Input: part model. Units: mm. Frame: model coordinates. Face numbers are marked on the shaded views. A direction names the side the tool comes from. Give positions to 0.01 mm unless a question says otherwise; leave off trailing zeros. Loops run counter-clockwise (first coordinate to the right, second up) from the corner with the lowest first, then second, coordinate; pieces in that order, holes last. Notation, with made-up numbers: (37, 40.25) -> (55, 40.25) arc R14 ccw to (55, 48.25) -> close; hole circle Ø11 at (-24, -9). An arc over 180 degrees is marked (long way). Answer as a JSON object with one key per item and string values. Group by question number.
```python
from build123d import *

# Parameters (mm, degrees)
F2_R     = 0.7
F3_DEPTH = 2.761
F4_R     = 0.25
F5_DEPTH = 0.751
F6_R     = 0.12


with BuildPart() as f1:
    # F0 (on Top) → F1 (revolve)
    with BuildSketch(Plane.XY):
        Polygon((0, 2.76), (0, 0), (1.065, 0), (1.065, 2.01), (2.75, 2.01), (2.75, 2.76), align=None)
    revolve(axis=Axis((0, 1.38, 0), (0, 1, 0)))

    # F2 (on face) → F3 (cut, through all)
    with BuildSketch(Plane.XZ):
        Circle(F2_R)
    extrude(amount=-F3_DEPTH, mode=Mode.SUBTRACT)

    # F4 (on face) → F5 (cut, through all)
    with BuildSketch(Plane.XZ.offset(-2.01)):
        with Locations((0, 2.12)):
            Circle(F4_R)
        with Locations((2.12, 0)):
            Circle(F4_R)
        with Locations((0, -2.12)):
            Circle(F4_R)
        with Locations((-2.12, 0)):
            Circle(F4_R)
    extrude(amount=-F5_DEPTH, mode=Mode.SUBTRACT)

    # F6
    f6_edges = [f1.edges().sort_by_distance(p)[0] for p in [
        (-2.75, 2.01, 0),
        (-1.065, 2.01, 0),
        (-1.065, 0, 0),
    ]]
    fillet(f6_edges, radius=F6_R)


solid = f1.part
```
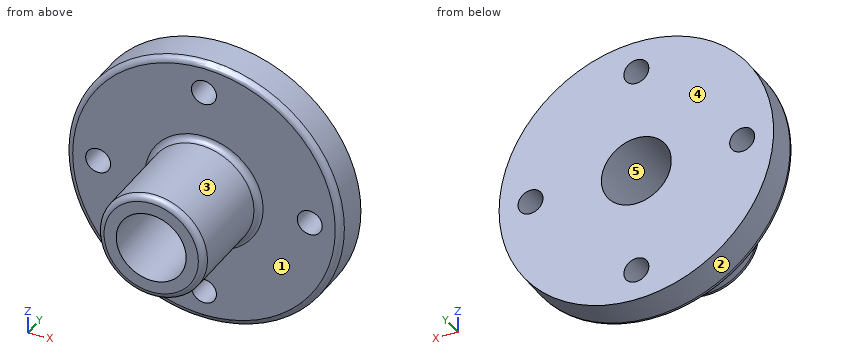
Q1. Pull-direction query (Z, two-part tool) for the marked faces 3, 4 and 5; classes: +Z half, -Z half, draft (parallel to the pull), parting line (faces both ways), or undercut.
Q2. Set-up query: the marked faces 1 and 2. Return all of +Z, -Z, +X, -X, +Y, -Y with unobstructed straight access to the full face (end or side cutting, diameter ignored); none if empty.
Q3. Section C-C on y = 1.05. Return the cut outline in (x, z) (3 decimals), then the cut area to 3 significant figures.
Q4. Ray query, probe 1 along Z at (x, y) = (0, 2.3); probe 2 along Z at (x, y) = (0, 1.3) (3 decimals); probe 3 along Y at (x, z) = (1.2, -2.35). Return the intervals inside material, ascending.
Q5. Section B-B on z = 0. Return the cut outline in (x, y) (3 decimals).
Q6. Section A-A on x = 0. Return the cut outline in (y, z) (3 decimals).
Numbers:
{
 "1": {"face 3": "parting line", "face 4": "draft", "face 5": "undercut"},
 "2": {"face 1": "-Y", "face 2": "+Y, -Y"},
 "3": {"outline": "circle Ø2.13 at (0, 0); hole circle Ø1.4 at (0, 0)", "area": "2.02 mm²"},
 "4": {"probe 1": "z = -2.75 to -2.37, -1.87 to -0.7, 0.7 to 1.87, 2.37 to 2.75", "probe 2": "z = -1.065 to -0.7, 0.7 to 1.065", "probe 3": "y = 2.01 to 2.76"},
 "5": {"outline": "(-2.75, 2.13) arc R0.12 ccw to (-2.63, 2.01) -> (-2.37, 2.01) -> (-2.37, 2.76) -> (-2.75, 2.76) -> close; (-1.87, 2.01) -> (-1.185, 2.01) arc R0.12 cw to (-1.065, 1.89) -> (-1.065, 0.12) arc R0.12 ccw to (-0.945, 0) -> (-0.7, 0) -> (-0.7, 2.76) -> (-1.87, 2.76) -> close; (0.7, 0) -> (0.945, 0) arc R0.12 ccw to (1.065, 0.12) -> (1.065, 1.89) arc R0.12 cw to (1.185, 2.01) -> (1.87, 2.01) -> (1.87, 2.76) -> (0.7, 2.76) -> close; (2.37, 2.01) -> (2.63, 2.01) arc R0.12 ccw to (2.75, 2.13) -> (2.75, 2.76) -> (2.37, 2.76) -> close"},
 "6": {"outline": "(0, -0.945) arc R0.12 ccw to (0.12, -1.065) -> (1.89, -1.065) arc R0.12 cw to (2.01, -1.185) -> (2.01, -1.87) -> (2.76, -1.87) -> (2.76, -0.7) -> (0, -0.7) -> close; (0, 0.7) -> (2.76, 0.7) -> (2.76, 1.87) -> (2.01, 1.87) -> (2.01, 1.185) arc R0.12 cw to (1.89, 1.065) -> (0.12, 1.065) arc R0.12 ccw to (0, 0.945) -> close; (2.01, -2.63) arc R0.12 ccw to (2.13, -2.75) -> (2.76, -2.75) -> (2.76, -2.37) -> (2.01, -2.37) -> close; (2.01, 2.37) -> (2.76, 2.37) -> (2.76, 2.75) -> (2.13, 2.75) arc R0.12 ccw to (2.01, 2.63) -> close"}
}
